```python
from build123d import *

# Parameters (mm, degrees)
F0_W     = 177.8
F0_H     = 127
F0_W_2   = 152.4
F0_H_2   = 101.6
F1_DEPTH = 76.2
F2_DEPTH = 38.1
F3_R     = 5.08


with BuildPart() as f1:
    # F0 (on Front) → F1 (new body)
    with BuildSketch(Plane.XZ):
        Rectangle(F0_W, F0_H)
        Rectangle(F0_W_2, F0_H_2, mode=Mode.SUBTRACT)
    extrude(amount=F1_DEPTH)

    # F0 (on Front) → F2 (join)
    with BuildSketch(Plane.XZ):
        Rectangle(F0_W_2, F0_H_2)
    extrude(amount=F2_DEPTH)

    # F3
    f3_edges = [f1.edges().sort_by_distance(p)[0] for p in [
        (-88.9, -76.2, 0),
        (0, -76.2, 63.5),
        (0, -76.2, -63.5),
        (88.9, -76.2, 0),
        (-76.2, -76.2, 0),
        (0, -76.2, 50.8),
        (76.2, -76.2, 0),
        (0, -76.2, -50.8),
        (0, -38.1, 50.8),
        (76.2, -57.15, 50.8),
        (76.2, -38.1, 0),
        (76.2, -57.15, -50.8),
        (0, -38.1, -50.8),
        (-76.2, -57.15, 50.8),
        (-76.2, -38.1, 0),
        (-76.2, -57.15, -50.8),
        (-88.9, -38.1, 63.5),
        (0, 0, -63.5),
        (-88.9, 0, 0),
        (-88.9, -38.1, -63.5),
        (88.9, -38.1, -63.5),
        (88.9, -38.1, 63.5),
        (88.9, 0, 0),
        (0, 0, 63.5),
    ]]
    fillet(f3_edges, radius=F3_R)


solid = f1.part
```
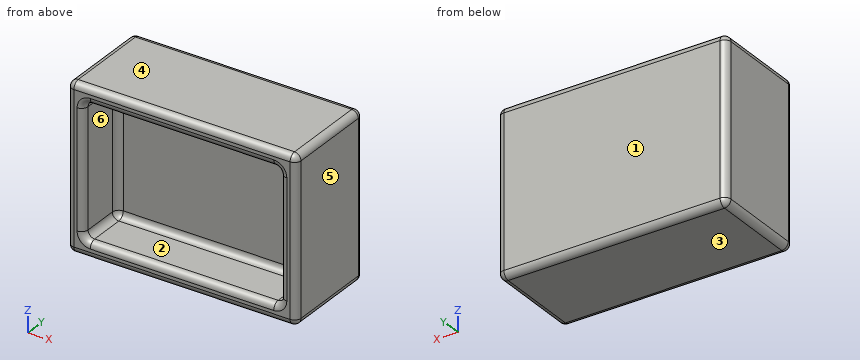
Can you work these out from the model? Positions are in its coordinate system, mm. Face numbers are marked on the shaded views. A direction names the side the tool comes from. Coordinates: 2 decimals unless noted, no trailing zeros. Loops run counter-clockwise (first coordinate to the right, second up) from the corner with the lowest first, then second, coordinate; pieces in that order, holes last.
1) Imagine slicing it at A-A on y = -55.5. List the corners of the cut face in (x, z) for me.
2) Imagine slicing it at B-B on z = -3.5. List the corners of the cut face in (x, y) for me, plus the area to 3 significant figures.
3) I need wall thicknesses on probe 1 along X at (y, z) = (-62, 1.5); probe 2 along Z at (x, y) = (13.5, -43); probe 3 along Y at (x, z) = (56, -35.5). Which ranges of each line are inside material? Lowest first, please.
4) For pin 1 (5 mm diameter, centred on x = -16.5, z = -9, fed in from -Y), with a flat end and sliding along its axis, tell me the tip position at first contact or that it passes through.
5) Imagine slicing it at C-C on x = -20. List the corners of the cut face in (y, z) for me, plus the area to 3 significant figures.
6) Thinking about a two-plate mould opening in Z: for the marked faces 3, 4, 5 and 6, which applies, pulls with the +Z half, pulls with the -Z half, needs draft (parallel to the pull), parting line crosses it, or undercut?
7) Which directions (+Z, -Z, +X, -X, +Y, -Y) give clear straight access to the entire face, cutting with the end or side of a thin tool? Please do the marked faces 1 and 2.
Completed:
1. outline: (-88.9, -58.42) arc R5.08 ccw to (-83.82, -63.5) - (83.82, -63.5) arc R5.08 ccw to (88.9, -58.42) - (88.9, 58.42) arc R5.08 ccw to (83.82, 63.5) - (-83.82, 63.5) arc R5.08 ccw to (-88.9, 58.42) - close; hole (-76.2, -45.72) arc R5.08 ccw to (-71.12, -50.8) - (71.12, -50.8) arc R5.08 ccw to (76.2, -45.72) - (76.2, 45.72) arc R5.08 ccw to (71.12, 50.8) - (-71.12, 50.8) arc R5.08 ccw to (-76.2, 45.72) - close
2. outline: (-88.9, -71.12) arc R5.08 ccw to (-83.82, -76.2) - (-81.28, -76.2) arc R5.08 ccw to (-76.2, -71.12) - (-76.2, -43.18) arc R5.08 cw to (-71.12, -38.1) - (71.12, -38.1) arc R5.08 cw to (76.2, -43.18) - (76.2, -71.12) arc R5.08 ccw to (81.28, -76.2) - (83.82, -76.2) arc R5.08 ccw to (88.9, -71.12) - (88.9, -5.08) arc R5.08 ccw to (83.82, 0) - (-83.82, 0) arc R5.08 ccw to (-88.9, -5.08) - close
2. area: 7,720 mm2
3. probe 1: x = -88.9 to -76.2, 76.2 to 88.9
3. probe 2: z = -63.5 to -50.8, 50.8 to 63.5
3. probe 3: y = -38.1 to 0
4. pin 1: stops at y = -38.1
5. outline: (-76.2, -58.42) arc R5.08 ccw to (-71.12, -63.5) - (-5.08, -63.5) arc R5.08 ccw to (0, -58.42) - (0, 58.42) arc R5.08 ccw to (-5.08, 63.5) - (-71.12, 63.5) arc R5.08 ccw to (-76.2, 58.42) - (-76.2, 55.88) arc R5.08 ccw to (-71.12, 50.8) - (-43.18, 50.8) arc R5.08 cw to (-38.1, 45.72) - (-38.1, -45.72) arc R5.08 cw to (-43.18, -50.8) - (-71.12, -50.8) arc R5.08 ccw to (-76.2, -55.88) - close
5. area: 5,780 mm2
6. face 3: pulls with the -Z half
6. face 4: pulls with the +Z half
6. face 5: needs draft
6. face 6: undercut
7. face 1: +Z, -Z, +X, -X, +Y
7. face 2: -Y
